```python
from build123d import *

# Parameters (mm, degrees)
SKETCH1_R           = 58
BOSS_EXTRUDE1_DEPTH = 8
SKETCH2_R           = 55
CUT_EXTRUDE1_DEPTH  = 5
SKETCH3_R           = 18.5
SKETCH3_R_2         = 9.5
BOSS_EXTRUDE2_DEPTH = 10
FILLET1_R           = 5
SKETCH4_R           = 13.315
SKETCH4_R_2         = 9.4
BOSS_EXTRUDE3_DEPTH = 17
CUT_EXTRUDE2_START  = -17
SKETCH5_R           = 9.4
CUT_EXTRUDE2_DEPTH  = 17


with BuildPart() as part:
    # Sketch1 → Boss-Extrude1 (new body)
    with BuildSketch(Plane.XY):
        Circle(SKETCH1_R)
    extrude(amount=BOSS_EXTRUDE1_DEPTH)

    # Sketch2 → Cut-Extrude1 (cut)
    with BuildSketch(Plane.XY.offset(8)):
        Circle(SKETCH2_R)
    extrude(amount=-CUT_EXTRUDE1_DEPTH, mode=Mode.SUBTRACT)

    # Sketch3 → Boss-Extrude2 (add)
    with BuildSketch(Plane.XY.offset(3)):
        Circle(SKETCH3_R)
        Circle(SKETCH3_R_2, mode=Mode.SUBTRACT)
    extrude(amount=BOSS_EXTRUDE2_DEPTH)

    # Fillet1
    fillet1_edges = [part.edges().sort_by_distance(p)[0] for p in [
        (-18.5, 0, 3),
    ]]
    fillet(fillet1_edges, radius=FILLET1_R)

    # Sketch4 → Boss-Extrude3 (add)
    with BuildSketch(Plane(origin=(0, 0, 0), x_dir=(-1, 0, 0), z_dir=(0, 0, -1))):
        with Locations(Location((0, 0, 0), (0, 0, 180))):
            Circle(SKETCH4_R)
        Circle(SKETCH4_R_2, mode=Mode.SUBTRACT)
    extrude(amount=BOSS_EXTRUDE3_DEPTH)

    # Sketch5 → Cut-Extrude2 (cut)
    with BuildSketch(Plane(origin=(0, 0, 0), x_dir=(-1, 0, 0), z_dir=(0, 0, -1)).offset(CUT_EXTRUDE2_START)):
        with Locations(Location((0, 0, 0), (0, 0, 180))):
            Circle(SKETCH5_R)
    extrude(amount=CUT_EXTRUDE2_DEPTH, mode=Mode.SUBTRACT)


solid = part.part
```
Here's how the part is built. I have some questions about the finished solid (model axes, mm). A direction names the side the tool comes from. Coordinates: 2 decimals unless noted, no trailing zeros. Write each loop counter-clockwise with the first axis right and the second up, starting at its lowest first coordinate (ties: lowest second). Pieces come first, ordered by that corner, then holes. Notation, with made-up numbers: (55.5, 39) -> (101.5, 39) arc R36 cw to (101.5, 77) -> close; hole circle Ø6 at (14.5, 3.25). An arc over 180 degrees is marked (long way). Use a Markdown table: item, result. Add a question column.
(1) If we section it at D-D, the plane x = 48.5: Write out the boundary of the cut face in (y, z).
(2) For faces 1 (the cylindrical face through (-11.923, -53.692, 5.535)), 2 (the cylindrical face through (-2.886, 12.998, -8.381)), which set-ups out of +Z, -Z, +X, -X, +Y, -Y let a thin tool reach every point of the face, with its end or its side?
(3) Please list where these lines run through material, in increasing order: line 1 (Y direction, x = 0, z = 1.6); line 2 (Y direction, x = 0, z = 4.65); line 3 (Y direction, x = 0, z = 5.5).
(4) I'm going to push flat-ended pins straight in: P1, Ø8, axis at x = 19, z = 2.5, coming from the +Y side; P2, Ø17, axis at x = 0, y = 0, coming from the -Z side; P3, Ø1.5, axis at x = 43, y = 22, coming from the +Z side; P4, Ø21, axis at x = -1.5, y = -3.5, coming from the +Z side. Where does each tip first touch, or does it pass through?
(5) If we section it at A-A, the plane y = 0: Write out the boundary of the cut face in (x, z) (3 decimals).
(6) We'd pull the mould along X, two halves only. Please class faces 3 (the flat face through (-1, -24, 3)), 4 (the cylindrical face through (-4.01, -18.06, 10.46)), 5 (the flat face through (8, -8, 13)): +X half, -X half, draft (parallel to the pull), parting line (faces both ways), or undercut.
(7) If we section it at C-C, the plane z = 9.5: Write out the boundary of the cut face in (x, y).
Outcome:
| question | item | result |
|---|---|---|
| 1 | outline | (-31.81, 0) -> (31.81, 0) -> (31.81, 8) -> (25.94, 8) -> (25.94, 3) -> (-25.94, 3) -> (-25.94, 8) -> (-31.81, 8) -> close |
| 2 | face 1 | +Z |
| 2 | face 2 | -Z |
| 3 | line 1 | y = -58 to -9.4, 9.4 to 58 |
| 3 | line 2 | y = -58 to -55, -19.79 to -9.5, 9.5 to 19.79, 55 to 58 |
| 3 | line 3 | y = -58 to -55, -19.17 to -9.5, 9.5 to 19.17, 55 to 58 |
| 4 | P1 | stops at y = 56.03 |
| 4 | P2 | passes through |
| 4 | P3 | stops at z = 3 |
| 4 | P4 | stops at z = 13 |
| 5 | outline | (-58, 0) -> (-13.315, 0) -> (-13.315, -17) -> (-9.4, -17) -> (-9.4, 3) -> (-9.5, 3) -> (-9.5, 13) -> (-18.5, 13) -> (-18.5, 8) arc R5 cw to (-23.5, 3) -> (-55, 3) -> (-55, 8) -> (-58, 8) -> close; (9.4, -17) -> (13.315, -17) -> (13.315, 0) -> (58, 0) -> (58, 8) -> (55, 8) -> (55, 3) -> (23.5, 3) arc R5 cw to (18.5, 8) -> (18.5, 13) -> (9.5, 13) -> (9.5, 3) -> (9.4, 3) -> close |
| 6 | face 3 | undercut |
| 6 | face 4 | parting line |
| 6 | face 5 | draft |
| 7 | outline | circle Ø37 at (0, 0); hole circle Ø19 at (0, 0) |
